The model under review builds one solid part; all positions refer to its coordinate system, in mm. Face numbers are marked on the shaded views. A direction names the side the tool comes from. Coordinates: 2 decimals unless noted, no trailing zeros. Write each loop counter-clockwise with the first axis right and the second up, starting at its lowest first coordinate (ties: lowest second). Pieces come first, ordered by that corner, then holes.
1) For P1, Ø1.5, axis at y = -7, z = 1, coming from the -X side; P2, Ø3, axis at x = 1.5, y = 3, coming from the +Z side; P3, Ø2, axis at x = 0.5, y = -15, coming from the -Z side, all flat-tipped, find the tip position at first contact; note any pin that passes through.
2) For line 1 (Z direction, x = 0.85, y = -9); line 2 (Y direction, x = -0.8, z = 2.7); line 3 (Z direction, x = 1.1, y = 3) (3 decimals), list the stretches that pass through material, from the lowest coordinate up.
3) Add section A-A, the plane y = -13. State the section outline as (x, z) points, then the cut area to 3 significant figures.
4) Machinability: for the marked faces 1, 2 and 3, which of the approach directions +Z, -Z, +X, -X, +Y, -Y give a long, thin tool a straight path to every point of the face, cutting with its end or side? Answer none if there is none.
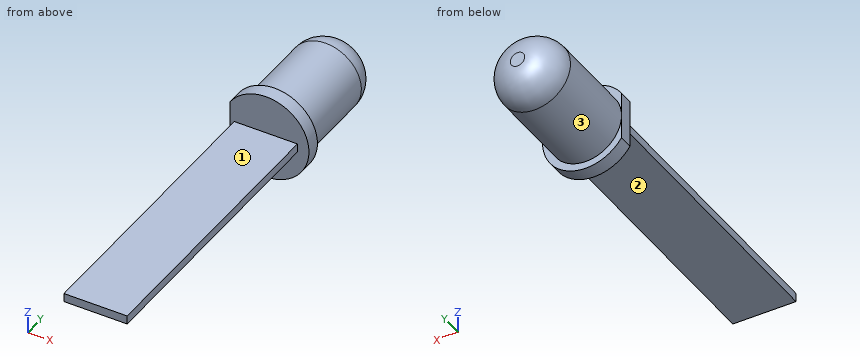
from build123d import *

# Parameters (mm, degrees)
SKETCH1_R           = 3
BOSS_EXTRUDE1_DEPTH = 1
SKETCH2_R           = 2.5
BOSS_EXTRUDE2_DEPTH = 8
FILLET1_R           = 2
SKETCH3_W           = 4.4
SKETCH3_H           = 0.6
BOSS_EXTRUDE3_DEPTH = 20
CUT_EXTRUDE1_START  = -2.5
SKETCH4_W           = 14.899802266
SKETCH4_H           = 5.02411501
CUT_EXTRUDE1_DEPTH  = 20


with BuildPart() as part:
    # Sketch1 → Boss-Extrude1 (new body)
    with BuildSketch(Plane(origin=(0, 0, 0), x_dir=(1, 0, 0), z_dir=(0, 1, 0))):
        with Locations(Location((0, 0, 0), (0, 0, 270))):
            Circle(SKETCH1_R)
    extrude(amount=BOSS_EXTRUDE1_DEPTH)

    # Sketch2 → Boss-Extrude2 (add)
    with BuildSketch(Plane(origin=(0, 1, 0), x_dir=(1, 0, 0), z_dir=(0, 1, 0))):
        with Locations(Location((0, 0, 0), (0, 0, 270))):
            Circle(SKETCH2_R)
    extrude(amount=BOSS_EXTRUDE2_DEPTH)

    # Fillet1
    fillet1_edges = [part.edges().sort_by_distance(p)[0] for p in [
        (0, 9, -2.5),
    ]]
    fillet(fillet1_edges, radius=FILLET1_R)

    # Sketch3 → Boss-Extrude3 (add)
    with BuildSketch(Plane.XZ):
        Rectangle(SKETCH3_W, SKETCH3_H)
    extrude(amount=BOSS_EXTRUDE3_DEPTH)

    # Sketch4 → Cut-Extrude1 (cut)
    with BuildSketch(Plane(origin=(0, 0, 0), x_dir=(0, 0, -1), z_dir=(1, 0, 0)).offset(CUT_EXTRUDE1_START)):
        Rectangle(SKETCH4_W, SKETCH4_H)
    extrude(amount=-CUT_EXTRUDE1_DEPTH, mode=Mode.SUBTRACT)


solid = part.part
Geometry results:
1. P1: stops at x = -2.2
1. P2: stops at z = 2.5
1. P3: stops at z = -0.3
2. line 1: z = -0.3 to 0.3
2. line 2: y = 0 to 1
2. line 3: z = -2.245 to 2.245
3. outline: (-2.2, -0.3) - (2.2, -0.3) - (2.2, 0.3) - (-2.2, 0.3) - close
3. area: 2.64 mm2
4. face 1: +Z, +X, -X, -Y
4. face 2: -Z, +X, -X, -Y
4. face 3: +Y
